The listing builds one solid part. Answer for the finished solid, in the listing's coordinates (mm). A direction names the side the tool comes from. Round coordinates to 2 decimals unless told otherwise and drop trailing zeros. Order: outer loops, then holes, each group sorted by start corner. A loop starts at its lowest first (then second) coordinate and runs counter-clockwise, first axis right, second up. Notation, with made-up numbers: (30.5, -37.5) -> (57.5, -37.5) arc R23 ccw to (57.5, -28.5) -> close; hole circle Ø7 at (-26.75, 16). An arc over 180 degrees is marked (long way). Answer in a Markdown table with one row per item. Add a question column.
```python
from build123d import *

# Parameters (mm, degrees)
SKETCH1_W           = 5
SKETCH1_H           = 75
BOSS_EXTRUDE1_DEPTH = 4
SKETCH2_W           = 3
SKETCH2_H           = 75
BOSS_EXTRUDE2_DEPTH = 1.65
SKETCH3_W           = 5
SKETCH3_H           = 75
BOSS_EXTRUDE3_DEPTH = 2
SKETCH4_R           = 1.5
CUT_EXTRUDE1_DEPTH  = 87.136650155


with BuildPart() as part:
    # Sketch1 → Boss-Extrude1 (new body)
    with BuildSketch(Plane.XY):
        with Locations((-28.5, -42.5)):
            Rectangle(SKETCH1_W, SKETCH1_H)
    extrude(amount=BOSS_EXTRUDE1_DEPTH)

    # Sketch2 → Boss-Extrude2 (add)
    with BuildSketch(Plane.XY.offset(4)):
        with Locations((-27.5, -42.5)):
            Rectangle(SKETCH2_W, SKETCH2_H)
    extrude(amount=BOSS_EXTRUDE2_DEPTH)

    # Sketch3 → Boss-Extrude3 (add)
    with BuildSketch(Plane.XY.offset(5.65)):
        with Locations((-28.5, -42.5)):
            Rectangle(SKETCH3_W, SKETCH3_H)
    extrude(amount=BOSS_EXTRUDE3_DEPTH)

    # Sketch4 → Cut-Extrude1 (cut, through all)
    with BuildSketch(Plane.XY.offset(7.65)):
        with Locations((-28.5, -73)):
            Circle(SKETCH4_R)
        with Locations((-28.5, -12)):
            Circle(SKETCH4_R)
    extrude(amount=-CUT_EXTRUDE1_DEPTH, mode=Mode.SUBTRACT)


solid = part.part
```
Item 1: Flat-ended cylindrical pins translate along their axes: P1, Ø0.5, axis at y = -8, z = 5, coming from the -X side; P2, Ø1.8, axis at y = -53.5, z = 5, coming from the -X side. Find the tip coordinate at first contact, or state that the pin passes through.
Item 2: A tool of negligible diameter and unlimited length cuts with its end or side. For faces 5 (the face through (-28.5, -5, 3.8)), 6 (the face through (-29, -8, 5)), from which of +Z, -Z, +X, -X, +Y, -Y can it reach the whole face along a straight path? Write none if from no direction.
Item 3: The part is cut by section C-C, the plane z = 1.75. Give the vertices of the cut face in (x, y).
Item 4: The part is cut by section B-B, the plane z = 5. Give the vertices of the cut face in (x, y).
Item 5: Find the intervals of material crossed by probe 1 along Y at (x, z) = (-28.5, 4.5); probe 2 along Z at (x, y) = (-29.5, -41); probe 3 along X at (y, z) = (-12, 2.5), in increasing order. Write a range as [from, to].
Item 6: For a pull along X with two mould halves and no side action, classify faces 1 (the face through (-26, -43, 4)), 2 (the face through (-29, -43, 5)), 3 (the face through (-27, -73, 4)), 4 (the face through (-28.5, -80, 3.8)) as released by +X, released by -X, zero draft, split by the parting line, or undercut.
Item 7: The part is cut by section D-D, the plane y = -40. Give the vertices of the cut face in (x, z), and give its area (4 significant figures).
Item 8: The part is cut by section A-A, the plane y = -12. Give the vertices of the cut face in (x, z), and give its area (4 significant figures).
Resolved:
| question | item | result |
|---|---|---|
| 1 | P1 | x = -29 |
| 1 | P2 | x = -31 |
| 2 | face 5 | +Z, -Z, +X, -X, +Y |
| 2 | face 6 | -X, +Y, -Y |
| 3 | outline | (-31, -80) -> (-26, -80) -> (-26, -5) -> (-31, -5) -> close; hole circle Ø3 at (-28.5, -73); hole circle Ø3 at (-28.5, -12) |
| 4 | outline | (-29, -80) -> (-26, -80) -> (-26, -5) -> (-29, -5) -> (-29, -10.59) arc R1.5 cw (long way) to (-29, -13.41) -> (-29, -71.59) arc R1.5 cw (long way) to (-29, -74.41) -> close |
| 5 | probe 1 | [-80, -74.5], [-71.5, -13.5], [-10.5, -5] |
| 5 | probe 2 | [0, 4], [5.65, 7.65] |
| 5 | probe 3 | [-31, -30], [-27, -26] |
| 6 | face 1 | released by +X |
| 6 | face 2 | released by -X |
| 6 | face 3 | undercut |
| 6 | face 4 | zero draft |
| 7 | outline | (-31, 0) -> (-26, 0) -> (-26, 7.65) -> (-31, 7.65) -> (-31, 5.65) -> (-29, 5.65) -> (-29, 4) -> (-31, 4) -> close |
| 7 | area | 34.95 mm2 |
| 8 | outline | (-31, 0) -> (-30, 0) -> (-30, 4) -> (-31, 4) -> close; (-31, 5.65) -> (-30, 5.65) -> (-30, 7.65) -> (-31, 7.65) -> close; (-27, 0) -> (-26, 0) -> (-26, 7.65) -> (-27, 7.65) -> close |
| 8 | area | 13.65 mm2 |
